Autodesk Inventor part; units mm, degrees
ref_plane "YZ Plane" through (0, 0, 0) normal (1, 0, 0) x (0, 1, 0)
ref_plane "XZ Plane" through (0, 0, 0) normal (0, 1, 0) x (-1, 0, 0)
ref_plane "XY Plane" through (0, 0, 0) normal (0, 0, 1) x (1, 0, 0)
sketch "Sketch1" plane through (0, 0, 0) normal (0, 0, 1) x (1, 0, 0)
  line L0 (0, 0) -> (-65, 0)
  line L1 (-65, 0) -> (-65, 65)
  line L2 (-65, 65) -> (0, 65)
  line L3 (0, 65) -> (0, 0)
  dimension "d4" = 65
  dimension "d5" = 65
extrude "Extrusion1" add sketch "Sketch1" along normal blind 6
sketch "Sketch2" plane through (0, 0, 6) normal (0, 0, 1) x (1, 0, 0)
  line L0 (-5, 5) -> (-60, 5)
  line L1 (-60, 5) -> (-60, 60)
  line L2 (-60, 60) -> (-5, 60)
  line L3 (-5, 60) -> (-5, 5)
  point P0 (0, 0)
  dimension "d8" = 55
  dimension "d9" = 55
extrude "Extrusion2" cut sketch "Sketch2" against normal blind 2
sketch "Sketch4" plane through (0, 0, 0) normal (0, 0, -1) x (-1, 0, 0)
  line L0 (32.5, 32.5) -> (29.7, 32.5)
  line L1 (29.7, 32.5) -> (29.7, 35.3)
  line L2 (29.7, 35.3) -> (32.5, 35.3)
  line L3 (32.5, 35.3) -> (32.5, 32.5)
  line L4 (29.7, 35.3) -> (35.3, 35.3)
  line L5 (35.3, 35.3) -> (35.3, 29.7)
  line L6 (35.3, 29.7) -> (29.7, 29.7)
  line L7 (29.7, 29.7) -> (29.7, 35.3)
  point P0 (0, 0)
  dimension "d30" = 2.8
  dimension "d31" = 2.8
  dimension "d32" = 5.6
  dimension "d33" = 5.6
extrude "Extrusion6" cut sketch "Sketch4" against normal blind 3
properties part number "Clip_MarkerHolderV1"
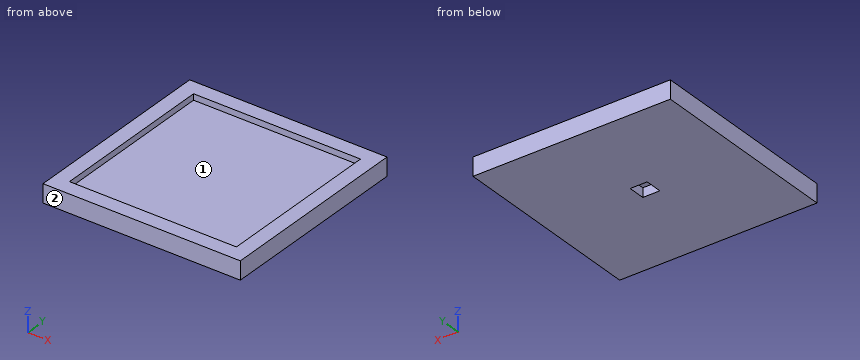
CAD build for the part. Positions are in the model's coordinates, mm. Face numbers are marked on the shaded views. A direction names the side the tool comes from. Round coordinates to 2 decimals unless told otherwise and drop trailing zeros. Order: outer loops, then holes, each group sorted by start corner. A loop starts at its lowest first (then second) coordinate and runs counter-clockwise, first axis right, second up. Notation, with made-up numbers: (66, -32) - (70, -32) arc R25 ccw to (70, -12) - close; hole circle Ø3 at (75, 64.5). An arc over 180 degrees is marked (long way). Answer as CSV lines item,"result". Start each with the question number.
1. Tool access for the marked faces 1 and 2: list every direction of +Z, -Z, +X, -X, +Y, -Y with a clear straight run to the whole face (end or side of a thin tool).
2. Saw through at D-D, the plane x = -33.5. Write the cut outline in (y, z), and give its area (3 significant figures).
3. Saw through at C-C, the plane y = 40. Write the cut outline in (x, z), and give its area (3 significant figures).
4. Saw through at A-A, the plane x = -52.5. Write the cut outline in (y, z).
5. Saw through at B-B, the plane y = 32. Write the cut outline in (x, z).
6. Pin check, flat tip, straight feed: pin 1 (4 mm diameter, centred on x = -12.5, y = 42, fed in from +Z). Stop position of the tip, or through.
7. Drill centre lines: L1, parallel to X at y = 6, z = 4.3; L2, parallel to Y at x = -58, z = 4.05; L3, parallel to Z at x = -40.5, y = 15.5. Where is each one in solid material? Low to high. Write a range as [from, to].
Model answer:
1,face 1,"+Z"
1,face 2,"+Z, -Z, +X, -X, -Y"
2,outline,"(0, 0) - (29.7, 0) - (29.7, 3) - (35.3, 3) - (35.3, 0) - (65, 0) - (65, 6) - (60, 6) - (60, 4) - (5, 4) - (5, 6) - (0, 6) - close"
2,area,"263 mm²"
3,outline,"(-65, 0) - (0, 0) - (0, 6) - (-5, 6) - (-5, 4) - (-60, 4) - (-60, 6) - (-65, 6) - close"
3,area,"280 mm²"
4,outline,"(0, 0) - (65, 0) - (65, 6) - (60, 6) - (60, 4) - (5, 4) - (5, 6) - (0, 6) - close"
5,outline,"(-65, 0) - (-35.3, 0) - (-35.3, 3) - (-29.7, 3) - (-29.7, 0) - (0, 0) - (0, 6) - (-5, 6) - (-5, 4) - (-60, 4) - (-60, 6) - (-65, 6) - close"
6,pin 1,"stops at z = 4"
7,L1,"x = [-65, -60], [-5, 0]"
7,L2,"y = [0, 5], [60, 65]"
7,L3,"z = [0, 4]"
